Autodesk Fusion 360 part; units mm, degrees
sketch "Sketch1" plane through (0, 0, 0) normal (0, 1, 0) x (1, 0, 0)
  line L0 (0, 0) -> (58.8, 0)
  line L1 (58.8, 0) -> (58.8, 75)
  line L2 (58.8, 75) -> (0, 75)
  line L3 (0, 75) -> (0, 0)
  dimension "d1" = 58.8
  dimension "d2" = 75
extrude "Extrude1" add sketch "Sketch1" along normal blind 3
sketch "Sketch2" plane through (0, 3, 0) normal (0, 1, 0) x (-1, 0, 0)
  line L0 (0, -75) -> (0, 0)
  line L1 (0, 0) -> (-58.8, 0)
  line L2 (-58.8, 0) -> (-58.8, -75)
  line L3 (-58.8, -75) -> (0, -75)
  line L4 (-10, -65) -> (-48.8, -65)
  line L5 (-48.8, -65) -> (-48.8, -10)
  line L6 (-48.8, -10) -> (-10, -10)
  line L7 (-10, -10) -> (-10, -65)
  dimension "d5" = 10
  dimension "d6" = 10
  dimension "d7" = 10
  dimension "d8" = 10
sketch "plate-2026-03-17T21_53_59.045Z" plane through (0, 3, 0) normal (0, 1, 0) x (0, 0, 1)
  line L0 (-44.8182, 45.8566) -> (-31.8182, 45.8566)
  line L1 (-44.8182, 31.8566) -> (-31.8182, 31.8566)
  line L2 (-45.3182, 45.3566) -> (-45.3182, 32.3566)
  line L3 (-31.3182, 45.3566) -> (-31.3182, 32.3566)
  arc A0 (-44.8182, 45.8566) -> (-45.3182, 45.3566) centre (-44.8182, 45.3566) ccw
  arc A1 (-31.3182, 45.3566) -> (-31.8182, 45.8566) centre (-31.8182, 45.3566) ccw
  arc A2 (-45.3182, 32.3566) -> (-44.8182, 31.8566) centre (-44.8182, 32.3566) ccw
  arc A3 (-31.8182, 31.8566) -> (-31.3182, 32.3566) centre (-31.8182, 32.3566) ccw
  line L4 (-25.7682, 45.8566) -> (-12.7682, 45.8566)
  line L5 (-25.7682, 31.8566) -> (-12.7682, 31.8566)
  line L6 (-26.2682, 45.3566) -> (-26.2682, 32.3566)
  line L7 (-12.2682, 45.3566) -> (-12.2682, 32.3566)
  arc A4 (-25.7682, 45.8566) -> (-26.2682, 45.3566) centre (-25.7682, 45.3566) ccw
  arc A5 (-12.2682, 45.3566) -> (-12.7682, 45.8566) centre (-12.7682, 45.3566) ccw
  arc A6 (-26.2682, 32.3566) -> (-25.7682, 31.8566) centre (-25.7682, 32.3566) ccw
  arc A7 (-12.7682, 31.8566) -> (-12.2682, 32.3566) centre (-12.7682, 32.3566) ccw
  line L8 (-44.8182, 26.8066) -> (-31.8182, 26.8066)
  line L9 (-44.8182, 12.8066) -> (-31.8182, 12.8066)
  line L10 (-45.3182, 26.3066) -> (-45.3182, 13.3066)
  line L11 (-31.3182, 26.3066) -> (-31.3182, 13.3066)
  arc A8 (-44.8182, 26.8066) -> (-45.3182, 26.3066) centre (-44.8182, 26.3066) ccw
  arc A9 (-31.3182, 26.3066) -> (-31.8182, 26.8066) centre (-31.8182, 26.3066) ccw
  arc A10 (-45.3182, 13.3066) -> (-44.8182, 12.8066) centre (-44.8182, 13.3066) ccw
  arc A11 (-31.8182, 12.8066) -> (-31.3182, 13.3066) centre (-31.8182, 13.3066) ccw
  line L12 (-25.7682, 26.8066) -> (-12.7682, 26.8066)
  line L13 (-25.7682, 12.8066) -> (-12.7682, 12.8066)
  line L14 (-26.2682, 26.3066) -> (-26.2682, 13.3066)
  line L15 (-12.2682, 26.3066) -> (-12.2682, 13.3066)
  arc A12 (-25.7682, 26.8066) -> (-26.2682, 26.3066) centre (-25.7682, 26.3066) ccw
  arc A13 (-12.2682, 26.3066) -> (-12.7682, 26.8066) centre (-12.7682, 26.3066) ccw
  arc A14 (-26.2682, 13.3066) -> (-25.7682, 12.8066) centre (-25.7682, 13.3066) ccw
  arc A15 (-12.7682, 12.8066) -> (-12.2682, 13.3066) centre (-12.7682, 13.3066) ccw
  line L16 (-47.8432, 10.2816) -> (-9.7432, 10.2816)
  line L17 (-47.8432, 48.3816) -> (-9.7432, 48.3816)
  line L18 (-47.8432, 10.2816) -> (-47.8432, 48.3816)
  line L19 (-9.7432, 10.2816) -> (-9.7432, 48.3816)
extrude "Extrude2" cut sketch "plate-2026-03-17T21_53_59.045Z" against normal blind 3 contours L0 L1 L2 L3 A0 A1 A2 A3 | L4 L5 L6 L7 A4 A5 A6 A7 | L8 L9 L10 L11 A8 A9 A10 A11 | L12 L13 L14 L15 A12 A13 A14 A15
sketch "Sketch4" plane through (0, 3, 0) normal (0, 1, 0) x (-1, 0, 0)
  line L0 (-12.5, -61.899) -> (-42.5, -61.899)
  line L1 (-42.5, -61.899) -> (-42.5, -49.899)
  line L2 (-42.5, -49.899) -> (-12.5, -49.899)
  line L3 (-12.5, -49.899) -> (-12.5, -61.899)
  line L4 (-10, -10) -> (-10, -65)
  dimension "d11" = 12
  dimension "d12" = 30
  dimension "d13" = 2.5
extrude "Extrude3" cut sketch "Sketch4" against normal blind 3
sketch "Sketch5" plane through (0, 3, 0) normal (0, 1, 0) x (-1, 0, 0)
  circle A0 centre (-5, -70) radius 1.45
  circle A1 centre (-5, -5) radius 1.45
  circle A2 centre (-53.8, -70) radius 1.45
  circle A3 centre (-53.8, -5) radius 1.45
  line L0 (-58.8, -75) -> (0, -75)
  line L1 (0, -75) -> (0, 0)
  line L2 (0, 0) -> (-58.8, 0)
  line L3 (-58.8, 0) -> (-58.8, -75)
  dimension "d16" = 2.9
  dimension "d17" = 2.9
  dimension "d18" = 2.9
  dimension "d19" = 2.9
  dimension "d20" = 5
  dimension "d21" = 5
  dimension "d22" = 5
  dimension "d23" = 5
  dimension "d24" = 5
  dimension "d25" = 5
  dimension "d26" = 5
  dimension "d27" = 5
extrude "Extrude4" cut sketch "Sketch5" against normal blind 3 contours A0 | A1 | A2 | A3
The listing builds one solid part. Answer for the finished solid, in the listing's coordinates (mm). A direction names the side the tool comes from. Round coordinates to 2 decimals unless told otherwise and drop trailing zeros. Order: outer loops, then holes, each group sorted by start corner. A loop starts at its lowest first (then second) coordinate and runs counter-clockwise, first axis right, second up. Notation, with made-up numbers: (10, 69.25) -> (69, 69.25) arc R19 cw to (69, 101.25) -> close; hole circle Ø4 at (58.25, 53.25). An arc over 180 degrees is marked (long way). One line per item, written item: value.
Item 1: For a pull along X with two mould halves and no side action, classify faces 3 (the flat face through (20, 2, -45.318)), 4 (the flat face through (29, 1, 0)), 5 (the flat face through (0, 1, -38)) as released by +X, released by -X, zero draft, split by the parting line, or undercut.
Taken from the geometry:
face 3: undercut
face 4: zero draft
face 5: released by -X
Item 2: For faces 1 (the flat face through (39, 2, -12.268)), 2 (the flat face through (29, 0, -38)), determine the directions among +Z, -Z, +X, -X, +Y, -Y from which every point of the face is accessible in a straight line to the end or side of a thin tool.
Taken from the geometry:
face 1: +Y, -Y
face 2: +Z, -Z, +X, -X, -Y
Item 3: Find section C-C, the plane x = 5. Give the vertices of the cut face in (y, z), then the cut area to 3 significant figures.
Taken from the geometry:
outline: (0, -75) -> (3, -75) -> (3, -71.45) -> (0, -71.45) -> close; (0, -68.55) -> (3, -68.55) -> (3, -6.45) -> (0, -6.45) -> close; (0, -3.55) -> (3, -3.55) -> (3, 0) -> (0, 0) -> close
area: 208 mm2
Item 4: Straight lines are drawn through the part: L1, parallel to Z at x = 45, y = 1.6; L2, parallel to X at y = 1.95, z = -22; L3, parallel to Z at x = 5, y = 2.35. For each, find the intervals that lie inside material, in ascending order.
Taken from the geometry:
L1: z = -75 to -45.32, -31.32 to -26.27, -12.27 to 0
L2: x = 0 to 12.81, 26.81 to 31.86, 45.86 to 58.8
L3: z = -75 to -71.45, -68.55 to -6.45, -3.55 to 0
Item 5: Find section D-D, the plane y = 2.5. State how many separate pieces and enclosed holes the cut face has, then the cut area to 3 significant figures.
Taken from the geometry:
separate pieces: 1
enclosed holes: 9
area: 3,240 mm2
Item 6: Find section A-A, the plane z = -21. Give the vertices of the cut face in (x, y).
Taken from the geometry:
outline: (0, 0) -> (12.81, 0) -> (12.81, 3) -> (0, 3) -> close; (26.81, 0) -> (31.86, 0) -> (31.86, 3) -> (26.81, 3) -> close; (45.86, 0) -> (58.8, 0) -> (58.8, 3) -> (45.86, 3) -> close
Item 7: Find section B-B, the plane x = 23. Give the vertices of the cut face in (y, z), then the cut area to 3 significant figures.
Taken from the geometry:
outline: (0, -75) -> (3, -75) -> (3, -61.9) -> (0, -61.9) -> close; (0, -49.9) -> (3, -49.9) -> (3, -45.32) -> (0, -45.32) -> close; (0, -31.32) -> (3, -31.32) -> (3, -26.27) -> (0, -26.27) -> close; (0, -12.27) -> (3, -12.27) -> (3, 0) -> (0, 0) -> close
area: 105 mm2
